Check sheet for the modelled part. Datum: model origin and axes. Units: mm. A direction names the side the tool comes from. Give positions to 0.01 mm unless a question says otherwise; leave off trailing zeros. Write each loop counter-clockwise with the first axis right and the second up, starting at its lowest first coordinate (ties: lowest second). Pieces come first, ordered by that corner, then holes.
from build123d import *

# Parameters (mm, degrees)
SKETCH1_R           = 2
BOSS_EXTRUDE1_DEPTH = 20
CUT_EXTRUDE1_DEPTH  = 1


with BuildPart() as part:
    # Sketch1 → Boss-Extrude1 (new body)
    with BuildSketch(Plane(origin=(0, 0, 0), x_dir=(1, 0, 0), z_dir=(0, 1, 0))):
        with Locations(Location((0, 0, 0), (0, 0, 270))):
            Circle(SKETCH1_R)
    extrude(amount=BOSS_EXTRUDE1_DEPTH)

    # Sketch3 → Revolve1 (revolve)
    with BuildSketch(Plane(origin=(0, 0, 0), x_dir=(0, 0, -1), z_dir=(1, 0, 0)), mode=Mode.PRIVATE) as revolve1_sk:
        Polygon((0, 20), (3.9, 20), (0, 16.1), align=None)
    revolve(revolve1_sk.sketch.rotate(Axis((0, 16.1, 0), (0, 1, 0)), 180), axis=Axis((0, 16.1, 0), (0, 1, 0)))

    # Sketch4 → Cut-Extrude1 (cut)
    with BuildSketch(Plane(origin=(0, 20, 0), x_dir=(1, 0, 0), z_dir=(0, 1, 0))):
        Polygon((0, 1.732050808), (-1.5, 0.866025404), (-1.5, -0.866025404), (0, -1.732050808), (1.5, -0.866025404), (1.5, 0.866025404), align=None)
    extrude(amount=-CUT_EXTRUDE1_DEPTH, mode=Mode.SUBTRACT)


solid = part.part
1) Draft check along X on faces 1 (the flat face through (-0.74, 19.507, -1.305)), 2 (the flat face through (0, 0, 0)), 3 (the cylindrical face through (-2, 9, 0)). Enter one of: +X half, -X half, draft (parallel to the pull), parting line (faces both ways), or undercut.
2) Sectioned sample at B-B on y = 11.5. Record the boundary of the cut face in (x, z), then the cut area to 3 significant figures.
3) Access from +Z, -Z, +X, -X, +Y, -Y to the whole of each face (thin tool, end or side, straight path). Record for faces 4 (the flat face through (0.74, 19.507, 1.305)), 5 (the flat face through (-2, 20, 0)).
4) Gauge pin test, flat ends, axial feed: pin 1 (1.5 mm diameter, centred on x = -2.5, y = 11, fed in from -Z); pin 2 (4 mm diameter, centred on y = 11.5, z = -2.5, fed in from -X); pin 3 (1.5 mm diameter, centred on y = 11, z = -0.5, fed in from +X). Record the tip position at first contact, or that the pin passes through.
5) Sectioned sample at A-A on z = 0. Record the boundary of the cut face in (x, y).
6) Scan lines: L1, parallel to X at y = 16.5, z = 0; L2, parallel to Y at x = -0.5, z = 0; L3, parallel to Z at x = 1.5, y = 9. Record each from-to range of solid material in increasing order.
Answers below:
1. face 1: undercut
1. face 2: draft
1. face 3: parting line
2. outline: circle Ø4 at (0, 0)
2. area: 12.6 mm2
3. face 4: +Y
3. face 5: +Z, -Z, +X, -X, +Y
4. pin 1: stops at z = -0.97
4. pin 2: stops at x = -1.94
4. pin 3: stops at x = 2
5. outline: (-3.9, 20) - (-2, 18.1) - (-2, 0) - (2, 0) - (2, 18.1) - (3.9, 20) - (1.5, 20) - (1.5, 19) - (-1.5, 19) - (-1.5, 20) - close
6. L1: x = -2 to 2
6. L2: y = 0 to 19
6. L3: z = -1.32 to 1.32
